Autodesk Inventor part; units mm, degrees
ref_plane "YZ Plane" through (0, 0, 0) normal (1, 0, 0) x (0, 1, 0)
ref_plane "XZ Plane" through (0, 0, 0) normal (0, 1, 0) x (-1, 0, 0)
ref_plane "XY Plane" through (0, 0, 0) normal (0, 0, 1) x (1, 0, 0)
sketch "Sketch1" plane through (0, 0, 0) normal (1, 0, 0) x (0, 1, 0)
  circle A0 centre (0, 0) radius 1.6256
  dimension "d0" = 3.2512
extrude "Extrusion1" add sketch "Sketch1" along normal blind 3.2512
thread "Thread1"
sketch "Sketch2" plane through (3.2512, 0, 0) normal (1, 0, 0) x (0, 0, -1)
  circle A0 centre (0, 0) radius 1.6256
extrude "Extrusion2" add sketch "Sketch2" along normal blind 3.2512
sketch "Sketch3" plane through (6.5024, 0, 0) normal (1, 0, 0) x (0, 0, -1)
  circle A0 centre (0, 0) radius 3.7786
extrude "Extrusion3" add sketch "Sketch3" along normal blind 3.2512
fillet "Fillet1" radius 1.5875 1 edges at (9.7536, 0, 3.7786)
sketch "Sketch4" plane through (9.7536, 0, 0) normal (1, 0, 0) x (0, 0, -1)
  circle A0 centre (0, 0) radius 2.1911
  line L0 (0, 2.1911) -> (2.0838, 0.6771)
  line L1 (2.0838, 0.6771) -> (1.2879, -1.7726)
  line L2 (1.2879, -1.7726) -> (-1.2879, -1.7726)
  line L3 (-1.2879, -1.7726) -> (-2.0838, 0.6771)
  line L4 (-2.0838, 0.6771) -> (0, 2.1911)
extrude "Extrusion4" cut sketch "Sketch4" against normal blind 2.2987 contours L1 L2 L3 L4 L0
chamfer "Chamfer1" distance 0.762 angle 45 1 edges at (0, -1.6256, 0)
properties part number "hex nut"
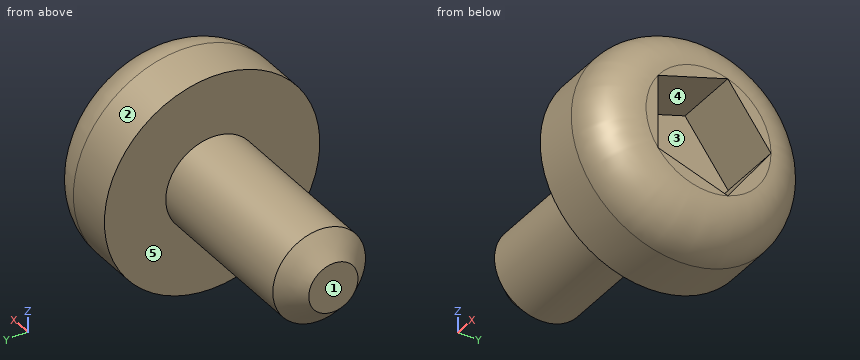
Design review of the part built by this model. Coordinates are the model's own, in mm. Face numbers are marked on the shaded views. A direction names the side the tool comes from. Give positions to 0.01 mm unless a question says otherwise; leave off trailing zeros. Write each loop counter-clockwise with the first axis right and the second up, starting at its lowest first coordinate (ties: lowest second). Pieces come first, ordered by that corner, then holes.
(1) Wall thickness on line 1 along X through (y, z) = (1.75, -0.5); line 2 along Z through (x, y) = (2.25, -0.5); line 3 along X through (y, z) = (2.5, 1.75): over which ranges is each line inside the solid? List them lowest first.
Checked values:
line 1: x = 6.5 to 7.45
line 2: z = -1.55 to 1.55
line 3: x = 6.5 to 9.5
(2) Clearance check with flat-ended pins moving along their axes: pin 1 Ø0.7 at (x, z) = (8, -0.5) entering from +Y; pin 2 Ø1.2 at (y, z) = (-0.5, 1) entering from +X; pin 3 Ø1.5 at (x, z) = (7, 2) entering from -Y. State where each tip first meets the part, or that it passes through.
Checked values:
pin 1: stops at y = 3.78
pin 2: stops at x = 7.45
pin 3: stops at y = -3.57
(3) Tool access review of the marked faces 4 and 5: name each direction out of +Z, -Z, +X, -X, +Y, -Y from which nothing blocks a thin tool from reaching the whole face with its end or side.
Checked values:
face 4: +X
face 5: -X
(4) Add section B-B (x = 1.25). Give the boundary of the cut face in (y, z), and give its area (3 significant figures).
Checked values:
outline: circle Ø3.25 at (0, 0)
area: 8.30 mm2
(5) Add section C-C (x = 7.25). Give the boundary of the cut face in (y, z).
Checked values:
outline: circle Ø7.56 at (0, 0)
(6) Mouldability with a two-part tool opening along Y and no side actions: class the marked faces 1, 2 and 3 as +Y half, -Y half, draft (parallel to the pull), parting line (faces both ways), or undercut.
Checked values:
face 1: draft
face 2: parting line
face 3: undercut
